Model file for the job. Use its own axes, mm. A direction names the side the tool comes from. Round coordinates to 2 decimals unless told otherwise and drop trailing zeros. Order: outer loops, then holes, each group sorted by start corner. A loop starts at its lowest first (then second) coordinate and runs counter-clockwise, first axis right, second up. Notation, with made-up numbers: (59, -9.5) - (66, -9.5) arc R26 cw to (66, 10.5) - close; hole circle Ø9 at (34, -25). An arc over 180 degrees is marked (long way). Answer as CSV lines item,"result". Start each with the question number.
1. Pull direction Z, two halves, no side cores. Call faces 3 (the face through (6, 0, 15)), 4 (the face through (3, 6, 30)), 5 (the face through (6, 6, 1)), 6 (the face through (3, 6, 0)): released by +Z, released by -Z, zero draft, split by the parting line, or undercut.
2. Band-saw the part on A-A on y = 15. List the corners of the cut face in (x, z), then the cut area to 3 significant figures.
3. Band-saw the part on C-C on z = 22.5. List the corners of the cut face in (x, y).
4. Pin check, flat tips, straight feed: pin 1 Ø3 at (y, z) = (15, 7.5) entering from -X; pin 2 Ø4.5 at (y, z) = (15, 22.5) entering from +X; pin 3 Ø6 at (x, z) = (8.5, 13) entering from +Y; pin 4 Ø4 at (y, z) = (13, 3) entering from +X. Stop position of each tip, or through.
5. Band-saw the part on B-B on x = 6. List the corners of the cut face in (y, z).
6. 3-axis set-ups, long thin cutter, end or side, ignore diameter. For faces 1 (the face through (-1.5, 3.5, 23.3)), 2 (the face through (0, 10, 15)): which of +Z, -Z, +X, -X, +Y, -Y reach the whole face in a straight line?
7. Wall check: line 1 along Z through (x, y) = (6, -1.75); line 2 along Y through (x, z) = (-2.15, 22.5); line 3 along Z through (x, y) = (1, 7.75). Give the ranges that are in metal, low to high. Write a range as [from, to].
8. Band-saw the part on D-D on x = 1. List the corners of the cut face in (y, z), then the cut area to 3 significant figures.
```python
from build123d import *

# Parameters (mm, degrees)
PROFILE_EXTRUDE_DEPTH     = 30
GUSSET_1_EXTRUDE_DEPTH    = 1.5
GUSSET_START              = 28.5
GUSSET_2_EXTRUDE_DEPTH    = 1.5
SOLENOID_MOUNTING_HOLES_D = 3.4
M3_MOUNTING_HOLES_D       = 3.4
CORNER_FILLETS_R          = 1.5


with BuildPart() as part:
    # Profile Sketch → Profile  Extrude (new body)
    with BuildSketch(Plane.XY):
        Polygon((0, 0), (0, 20), (-3, 20), (-3, -3), (12, -3), (12, 0), align=None)
    extrude(amount=PROFILE_EXTRUDE_DEPTH)

    # Gusset Sketch → Gusset 1 Extrude (add)
    with BuildSketch(Plane.XY):
        Polygon((0, 0), (12, 0), (0, 12), align=None)
    extrude(amount=GUSSET_1_EXTRUDE_DEPTH)

    # Gusset Sketch<2> → Gusset 2 Extrude (add)
    with BuildSketch(Plane.XY.offset(GUSSET_START)):
        Polygon((0, 0), (12, 0), (0, 12), align=None)
    extrude(amount=GUSSET_2_EXTRUDE_DEPTH)

    # Solenoid Mounting Holes (through all)
    with Locations(Plane(origin=(0, 0, 0), x_dir=(0, 0, -1), z_dir=(1, 0, 0))):
        with Locations((-7.5, 15), (-22.5, 15), (-22.5, 5), (-7.5, 5)):
            Hole(SOLENOID_MOUNTING_HOLES_D / 2)

    # M3 Mounting Holes (through all)
    with Locations(Plane(origin=(0, 0, 0), x_dir=(1, 0, 0), z_dir=(0, 1, 0))):
        with Locations((6, -22.5), (6, -7.5)):
            Hole(M3_MOUNTING_HOLES_D / 2)

    # Corner Fillets
    corner_fillets_edges = [part.edges().sort_by_distance(p)[0] for p in [
        (-1.5, 20, 30),
        (-1.5, 20, 0),
    ]]
    fillet(corner_fillets_edges, radius=CORNER_FILLETS_R)


solid = part.part
```
Reply:
1,face 3,"undercut"
1,face 4,"released by +Z"
1,face 5,"zero draft"
1,face 6,"released by -Z"
2,outline,"(-3, 0) - (0, 0) - (0, 5.8) - (-3, 5.8) - close; (-3, 9.2) - (0, 9.2) - (0, 20.8) - (-3, 20.8) - close; (-3, 24.2) - (0, 24.2) - (0, 30) - (-3, 30) - close"
2,area,"69.6 mm2"
3,outline,"(-3, -3) - (4.3, -3) - (4.3, 0) - (0, 0) - (0, 3.3) - (-3, 3.3) - close; (-3, 6.7) - (0, 6.7) - (0, 13.3) - (-3, 13.3) - close; (-3, 16.7) - (0, 16.7) - (0, 20) - (-3, 20) - close; (7.7, -3) - (12, -3) - (12, 0) - (7.7, 0) - close"
4,pin 1,"passes through"
4,pin 2,"stops at x = 0"
4,pin 3,"stops at y = 0"
4,pin 4,"stops at x = 0.32"
5,outline,"(-3, 0) - (6, 0) - (6, 1.5) - (0, 1.5) - (0, 5.8) - (-3, 5.8) - close; (-3, 9.2) - (0, 9.2) - (0, 20.8) - (-3, 20.8) - close; (-3, 24.2) - (0, 24.2) - (0, 28.5) - (6, 28.5) - (6, 30) - (-3, 30) - close"
6,face 1,"+X, -X"
6,face 2,"+X, +Y"
7,line 1,"z = [0, 5.8], [9.2, 20.8], [24.2, 30]"
7,line 2,"y = [-3, 3.3], [6.7, 13.3], [16.7, 20]"
7,line 3,"z = [0, 1.5], [28.5, 30]"
8,outline,"(-3, 0) - (11, 0) - (11, 1.5) - (0, 1.5) - (0, 28.5) - (11, 28.5) - (11, 30) - (-3, 30) - close"
8,area,"123 mm2"
